Part print with two shaded views. Sizes in mm from the minimum x, y, z corner. Give positions to 0.01 mm unless a question says otherwise; leave off trailing zeros. Write each loop counter-clockwise with the first axis right and the second up, starting at its lowest first coordinate (ties: lowest second). Pieces come first, ordered by that corner, then holes. Notation, with made-up numbers: (88.5, 66) -> (111.5, 66) arc R36 ccw to (111.5, 105) -> close; hole circle Ø1 at (-13.75, -16). An arc over 180 degrees is marked (long way). Write item = value, one per line. Start each with the question number.
Q1. Saw through at B-B, the plane z = 2.2. List the corners of the cut face in (x, y), then the cut area to 3 significant figures.
Q2. Drop flat-ended pins along their axis: P1, Ø0.9, axis at x = 35.5, z = 1.5, coming from the +Y side; P2, Ø1.5, axis at x = 36, z = 1, coming from the -Y side; P3, Ø0.9, axis at y = 34, z = 1.5, coming from the +X side. Give the stop position or say it passes through.
Q3. Wall check: line 1 (X direction, y = 5.5, z = 1.3); line 2 (Y direction, x = 20.5, z = 1.2); line 3 (X direction, y = 29.5, z = 0.7). Give the ranges that are in metal, low to high.
Q4. Saw through at A-A, the plane x = 21.5. List the corners of the cut face in (y, z), then the cut area to 3 significant figures.
Q5. Saw through at C-C, the plane y = 38. List the corners of the cut face in (x, z), then the cut area to 3 significant figures.
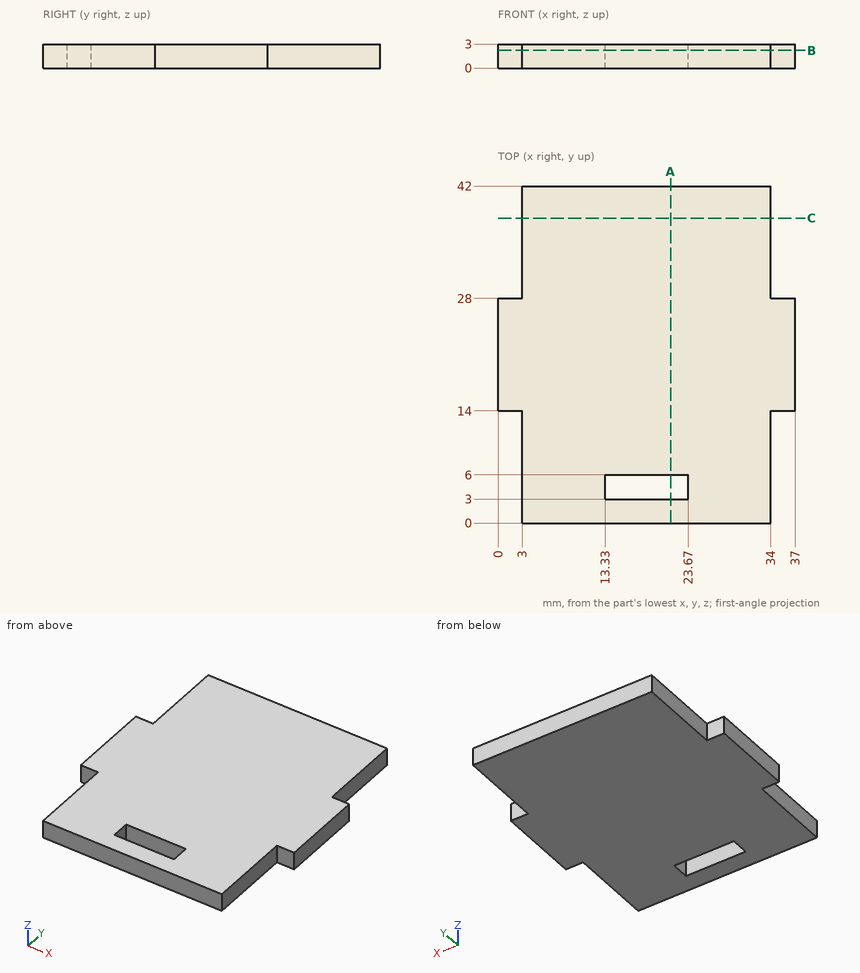
Report:
q1.outline = (0, 14) -> (3, 14) -> (3, 0) -> (34, 0) -> (34, 14) -> (37, 14) -> (37, 28) -> (34, 28) -> (34, 42) -> (3, 42) -> (3, 28) -> (0, 28) -> close; hole (13.33, 3) -> (23.67, 3) -> (23.67, 6) -> (13.33, 6) -> close
q1.area = 1,350 mm2
q2.P1 = 28
q2.P2 = 14
q2.P3 = 34
q3.line_1 = 3 to 13.33, 23.67 to 34
q3.line_2 = 0 to 3, 6 to 42
q3.line_3 = 3 to 34
q4.outline = (0, 0) -> (3, 0) -> (3, 3) -> (0, 3) -> close; (6, 0) -> (42, 0) -> (42, 3) -> (6, 3) -> close
q4.area = 117 mm2
q5.outline = (3, 0) -> (34, 0) -> (34, 3) -> (3, 3) -> close
q5.area = 93.0 mm2
